Model file for the job. Use its own axes, mm. A direction names the side the tool comes from. Give positions to 0.01 mm unless a question says otherwise; leave off trailing zeros. Loops run counter-clockwise (first coordinate to the right, second up) from the corner with the lowest first, then second, coordinate; pieces in that order, holes last. Notation, with made-up numbers: (57, -5.75) - (80, -5.75) arc R11 ccw to (80, 15.25) - close; hole circle Ø1 at (-36.5, -16.5). An arc over 180 degrees is marked (long way). Use a Markdown table: item, result.
from build123d import *

# Parameters (mm, degrees)
SKETCH1_W           = 100
SKETCH1_H           = 100
BOSS_EXTRUDE1_DEPTH = 1000
SKETCH6_W           = 50
SKETCH6_H           = 50
CUT_EXTRUDE1_DEPTH  = 1000
LPATTERN1_START     = 4.926108374
LPATTERN1_DEPTH     = 50


# Read off the part's stored shape, not the designer's step: LPattern1
with BuildPart() as part:
    # Sketch1 → Boss-Extrude1 (new body)
    with BuildSketch(Plane.XY):
        with Locations((-3.9408867, 4.926108374)):
            Rectangle(SKETCH1_W, SKETCH1_H)
    extrude(amount=-BOSS_EXTRUDE1_DEPTH)

    # Sketch6 → Cut-Extrude1 (cut, along a direction that is not the sketch's normal)
    with BuildSketch(Plane(origin=(46.0591133, 0, 0), x_dir=(0, 0, -1), z_dir=(1, 0, 0))):
        with Locations((75, 29.926108374)):
            Rectangle(SKETCH6_W, SKETCH6_H)
    extrude(amount=-CUT_EXTRUDE1_DEPTH, dir=(0.7071067811865516, 0, 0.7071067811865435), mode=Mode.SUBTRACT)

    # LPattern1 outline → LPattern1 (cut)
    with BuildSketch(Plane(origin=(0, 0, 0), x_dir=(1, 0, 0), z_dir=(0, 1, 0)).offset(LPATTERN1_START)):
        Polygon((-53.9408867, 100), (-53.9408867, 50), (-3.9408867, 0), (46.0591133, 0), align=None)
        Polygon((-53.9408867, 300), (-53.9408867, 250), (46.0591133, 150), (46.0591133, 200), align=None)
        Polygon((-53.9408867, 400), (-53.9408867, 350), (46.0591133, 250), (46.0591133, 300), align=None)
        Polygon((-53.9408867, 500), (-53.9408867, 450), (46.0591133, 350), (46.0591133, 400), align=None)
        Polygon((-53.9408867, 600), (-53.9408867, 550), (46.0591133, 450), (46.0591133, 500), align=None)
        Polygon((-53.9408867, 700), (-53.9408867, 650), (46.0591133, 550), (46.0591133, 600), align=None)
        Polygon((-53.9408867, 800), (-53.9408867, 750), (46.0591133, 650), (46.0591133, 700), align=None)
        Polygon((-53.9408867, 900), (-53.9408867, 850), (46.0591133, 750), (46.0591133, 800), align=None)
        Polygon((-53.9408867, 1000), (-53.9408867, 950), (46.0591133, 850), (46.0591133, 900), align=None)
        Polygon((46.0591133, 1000), (-3.9408867, 1000), (46.0591133, 950), align=None)
    extrude(amount=LPATTERN1_DEPTH, mode=Mode.SUBTRACT)


solid = part.part
(1) Pin check, flat tip, straight feed: P1, Ø15, axis at x = 29, z = -981, coming from the +Y side. Stop position of the tip, or through.
Computed:
| item | result |
|---|---|
| P1 | y = 4.93 |
(2) Drill centre lines: probe 1 along Y at (x, z) = (-38, -457); probe 2 along X at (y, z) = (34, -541.5); probe 3 along X at (y, z) = (21, -434). Where is each one in solid material? Low to high. Write a range as [from, to].
Computed:
| item | result |
|---|---|
| probe 1 | [-45.07, 4.93] |
| probe 2 | [-53.94, -45.44], [4.56, 46.06] |
| probe 3 | [-53.94, -37.94], [12.06, 46.06] |
(3) Slice it at A-A, the plane y = 32. Count the separate pieces of the cut face and the enclosed holes in it, plus the area to 3 significant figures.
Computed:
| item | result |
|---|---|
| separate pieces | 11 |
| enclosed holes | 0 |
| area | 50,000 mm² |
(4) 3-axis set-ups, long thin cutter, end or side, ignore diameter. For faces 4 (the flat face through (-8, 4.926, -825)), 5 (the flat face through (-4, 54.926, -169)), 6 (the flat face through (32, 4.926, -986)): which of +Z, -Z, +X, -X, +Y, -Y reach the whole face in a straight line?
Computed:
| item | result |
|---|---|
| face 4 | +Y |
| face 5 | +Z, -Z, +X, -X, +Y |
| face 6 | -Z, +X, +Y |
(5) Mould opens along Z. For faces 1 (the flat face through (20.71, 29.58, -975.35)), 2 (the flat face through (-4.64, 29.58, -400.7)), 3 (the flat face through (-4, 54.926, -769)) say: pulls with the +Z half, pulls with the -Z half, needs draft (parallel to the pull), parting line crosses it, or undercut.
Computed:
| item | result |
|---|---|
| face 1 | pulls with the -Z half |
| face 2 | undercut |
| face 3 | needs draft |
(6) Slice it at B-B, the plane z = -585. Write the cut outline in (x, y), plus the area to 3 significant figures.
Computed:
| item | result |
|---|---|
| outline | (-53.94, -45.07) - (46.06, -45.07) - (46.06, 4.93) - (11.06, 4.93) - (11.06, 54.93) - (-38.94, 54.93) - (-38.94, 4.93) - (-53.94, 4.93) - close |
| area | 7,500 mm² |
